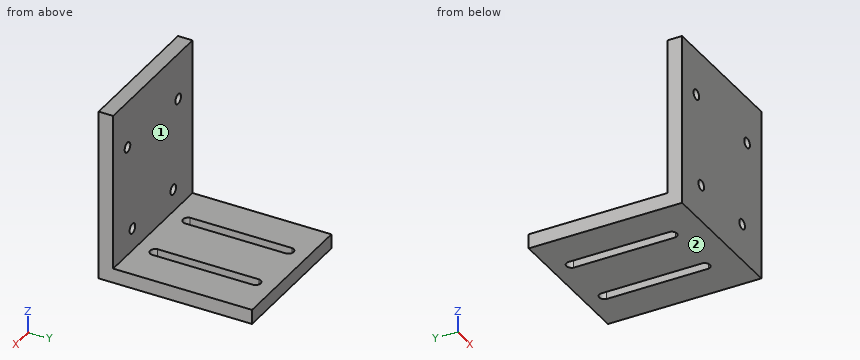
from build123d import *

# Parameters (mm, degrees)
SKETCH1_W                = 68.072
SKETCH1_H                = 76.327
BOSS_EXTRUDE1_DEPTH      = 63.0174
SKETCH2_W                = 69.8754
SKETCH2_H                = 61.6204
CUT_EXTRUDE1_DEPTH       = 113.452363516
CUT_EXTRUDE2_DEPTH       = 101.05830175
CUT_EXTRUDE3_DEPTH       = 105.665673231
M4_CLEARANCE_HOLE1_D     = 4.445
M4_CLEARANCE_HOLE1_DEPTH = 68.072


with BuildPart() as part:
    # Sketch1 → Boss-Extrude1 (new body)
    with BuildSketch(Plane(origin=(-15.262172061, 0, 0), x_dir=(0, -1, 0), z_dir=(-1, 0, 0))):
        with Locations((19.335625687, 38.1635)):
            Rectangle(SKETCH1_W, SKETCH1_H)
    extrude(amount=-BOSS_EXTRUDE1_DEPTH)

    # Sketch2 → Cut-Extrude1 (cut, through all)
    with BuildSketch(Plane(origin=(47.755227939, 0, 0), x_dir=(0, 0, -1), z_dir=(1, 0, 0))):
        with Locations((-41.3893, -16.109825687)):
            Rectangle(SKETCH2_W, SKETCH2_H)
    extrude(amount=-CUT_EXTRUDE1_DEPTH, mode=Mode.SUBTRACT)

    # Sketch3 → Cut-Extrude2 (cut, through all)
    with BuildSketch(Plane.XY.offset(6.4516)):
        with BuildLine():
            Line((5.464227939, -38.893127295), (5.464227939, 6.317876942))
            ThreePointArc((5.464227939, 6.317876942), (3.187772185, 8.223345793), (0.892227939, 6.340916789))
            Line((0.892227939, 6.340916789), (0.892227939, -38.916167142))
            ThreePointArc((0.892227939, -38.916167142), (3.187772185, -40.798596146), (5.464227939, -38.893127295))
        make_face()
    extrude(amount=-CUT_EXTRUDE2_DEPTH, mode=Mode.SUBTRACT)

    # Sketch4 → Cut-Extrude3 (cut, through all)
    with BuildSketch(Plane(origin=(0, 0, 0), x_dir=(-1, 0, 0), z_dir=(0, 0, -1))):
        with BuildLine():
            Line((-27.028827939, -38.893127295), (-27.028827939, 6.317876942))
            ThreePointArc((-27.028827939, 6.317876942), (-29.305283692, 8.223345793), (-31.600827939, 6.340916789))
            Line((-31.600827939, 6.340916789), (-31.600827939, -38.916167142))
            ThreePointArc((-31.600827939, -38.916167142), (-29.305283692, -40.798596146), (-27.028827939, -38.893127295))
        make_face()
    extrude(amount=-CUT_EXTRUDE3_DEPTH, mode=Mode.SUBTRACT)

    # M4 Clearance Hole1
    with Locations(Plane.XZ.offset(53.371625687)):
        with Locations((32.493055877, 16.408909131), (0, 16.408909131), (36.391998544, 55.735080284), (-3.898942667, 55.735080284)):
            Hole(M4_CLEARANCE_HOLE1_D / 2, depth=M4_CLEARANCE_HOLE1_DEPTH)


solid = part.part
Build history of the part. All positions in model axes, mm. Face numbers are marked on the shaded views. A direction names the side the tool comes from. Give positions to 0.01 mm unless a question says otherwise; leave off trailing zeros. Order: outer loops, then holes, each group sorted by start corner. A loop starts at its lowest first (then second) coordinate and runs counter-clockwise, first axis right, second up. Notation, with made-up numbers: M 54,82 L 102,82 A33 ccw 102,111 Z; hole C 82,59.25 d10. An arc over 180 degrees is marked long. Put each result on its own line as item: value.
Item 1: Slice it at C-C, the plane z = 46. Write the cut outline in (x, y).
From the geometry:
outline: M -15.26,-53.37 L 47.76,-53.37 L 47.76,-46.92 L -15.26,-46.92 Z
Item 2: Flat gauge pins, fed straight in: pin 1 Ø5 at (x, z) = (0, 16.41) entering from +Y; pin 2 Ø7 at (x, z) = (36.39, 55.74) entering from -Y. Where does each tip first touch, or does it go through?
From the geometry:
pin 1: stops at y = -46.92
pin 2: stops at y = -53.37
Item 3: 3-axis set-ups, long thin cutter, end or side, ignore diameter. For the marked faces 1 and 2: which of +Z, -Z, +X, -X, +Y, -Y reach the whole face in a straight line?
From the geometry:
face 1: +Z, +X, -X, +Y
face 2: -Z, +X, -X, +Y, -Y
Item 4: Probe line 1 (X direction, y = 4, z = 4.5); line 2 (Z direction, x = 0, y = -48.5); line 3 (Z direction, x = -1, y = -5). List the from-to ranges inside material, lowest first. Write a range as [from, to].
From the geometry:
line 1: x = [-15.26, 0.89], [5.46, 27.03], [31.6, 47.76]
line 2: z = [0, 14.19], [18.63, 76.33]
line 3: z = [0, 6.45]
Item 5: Slice it at B-B, the plane x = 22.5. Write the cut outline in (y, z).
From the geometry:
outline: M -53.37,0 L 14.7,0 L 14.7,6.45 L -46.92,6.45 L -46.92,76.33 L -53.37,76.33 Z
Item 6: Slice it at A-A, the plane y = -2. Write the cut outline in (x, z), plus the area to 3 significant figures.
From the geometry:
outline: M -15.26,0 L 0.89,0 L 0.89,6.45 L -15.26,6.45 Z; M 5.46,0 L 27.03,0 L 27.03,6.45 L 5.46,6.45 Z; M 31.6,0 L 47.76,0 L 47.76,6.45 L 31.6,6.45 Z
area: 348 mm2
